from build123d import *

# Parameters (mm, degrees)
SKETCH8_R           = 2.275
BOSS_EXTRUDE4_DEPTH = 4
SKETCH9_W           = 5
SKETCH9_H           = 6
BOSS_EXTRUDE5_DEPTH = 0.75
SKETCH10_R          = 1
BOSS_EXTRUDE6_DEPTH = 3
CUT_EXTRUDE2_DEPTH  = 1.5


with BuildPart() as part:
    # Sketch8 → Boss-Extrude4 (new body)
    with BuildSketch(Plane(origin=(0, 0, 0), x_dir=(1, 0, 0), z_dir=(0, 1, 0))):
        Circle(SKETCH8_R)
    extrude(amount=BOSS_EXTRUDE4_DEPTH)

    # Sketch9 → Boss-Extrude5 (add)
    with BuildSketch(Plane(origin=(0, 4, 0), x_dir=(1, 0, 0), z_dir=(0, 1, 0))):
        Rectangle(SKETCH9_W, SKETCH9_H)
    extrude(amount=BOSS_EXTRUDE5_DEPTH)

    # Sketch10 → Boss-Extrude6 (add, symmetric)
    with BuildSketch(Plane.XY):
        with BuildLine():
            Line((-2.896323692, 6.218137436), (-2.5, 4.75))
            Line((-2.5, 4.75), (2.5, 4.75))
            Line((2.5, 4.75), (2.896323692, 6.218137436))
            ThreePointArc((2.896323692, 6.218137436), (0, 10), (-2.896323692, 6.218137436))
        make_face()
        with Locations((0, 7)):
            Circle(SKETCH10_R, mode=Mode.SUBTRACT)
    extrude(amount=BOSS_EXTRUDE6_DEPTH, both=True)

    # Sketch11 → Cut-Extrude2 (cut, symmetric)
    with BuildSketch(Plane.XY):
        with BuildLine():
            Line((-0.119661192, 4.803256683), (-17.5, 5.75))
            Line((-17.5, 5.75), (-17.5, 11.234268724))
            Line((-17.5, 11.234268724), (17.5, 11.234268724))
            Line((17.5, 11.234268724), (17.5, 5.75))
            Line((17.5, 5.75), (0.119661192, 4.803256683))
            ThreePointArc((0.119661192, 4.803256683), (0, 4.8), (-0.119661192, 4.803256683))
        make_face()
    extrude(amount=CUT_EXTRUDE2_DEPTH, both=True, mode=Mode.SUBTRACT)


solid = part.part
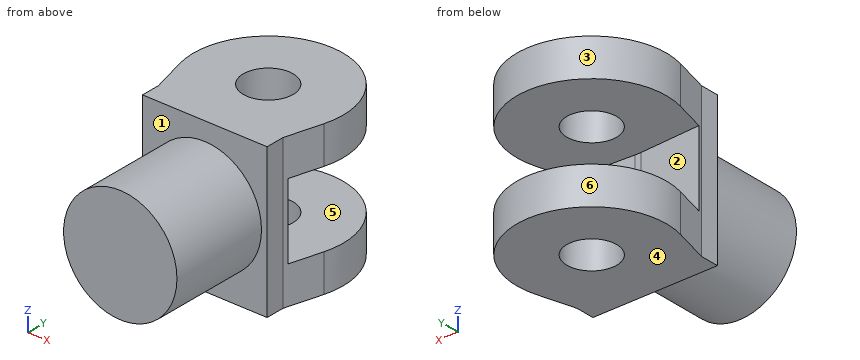
Read the model definition and answer for the solid it produces. Units are mm, in the model's axes. Face numbers are marked on the shaded views. A direction names the side the tool comes from. Coordinates: 2 decimals unless noted, no trailing zeros. Write each loop counter-clockwise with the first axis right and the second up, starting at its lowest first coordinate (ties: lowest second). Pieces come first, ordered by that corner, then holes. Notation, with made-up numbers: (86, 30) - (99, 30) arc R12 ccw to (99, 40) - close; hole circle Ø4 at (53, 34.25). An arc over 180 degrees is marked (long way). One line per question, with ' | ' between items.
Q1. Find section B-B, the plane x = 0. Write down the section's boundary in (y, z) (3 decimals).
Result set:
outline: (0, -2.275) - (4, -2.275) - (4, -3) - (6, -3) - (6, -1.5) - (4.8, -1.5) - (4.8, 1.5) - (6, 1.5) - (6, 3) - (4, 3) - (4, 2.275) - (0, 2.275) - close; (8, -3) - (10, -3) - (10, -1.5) - (8, -1.5) - close; (8, 1.5) - (10, 1.5) - (10, 3) - (8, 3) - close
Q2. Find section C-C, the plane z = 0. Write down the section's boundary in (x, y) (3 decimals).
Result set:
outline: (-2.55, 4.936) - (-2.5, 4.75) - (-2.5, 4) - (-2.275, 4) - (-2.275, 0) - (2.275, 0) - (2.275, 4) - (2.5, 4) - (2.5, 4.75) - (2.55, 4.936) - (0.12, 4.803) arc R2.2 cw to (-0.12, 4.803) - close
Q3. Each of these flat-tipped pins is pushed along its axis until it touches: P1, Ø3, axis at y = 2, z = 0.5, coming from the -X side (3 decimals); P2, Ø1.2, axis at x = 0, y = 7, coming from the +Z side; P3, Ø0.8, axis at y = 4.5, z = -1, coming from the -X side. Where does it stop, or does it pass through?
Result set:
P1: x = -2.275 | P2: through | P3: x = -2.54
Q4. Find section D-D, the plane y = 9. Write down the section's boundary in (x, z), plus the area to 3 significant figures.
Result set:
outline: (-2.24, -3) - (2.24, -3) - (2.24, -1.5) - (-2.24, -1.5) - close; (-2.24, 1.5) - (2.24, 1.5) - (2.24, 3) - (-2.24, 3) - close | area: 13.4 mm^2
Q5. For the marked faces 1, 2 and 3, determine the directions among +Z, -Z, +X, -X, +Y, -Y from which every point of the face is accessible in a straight line to the end or side of a thin tool.
Result set:
face 1: -Y | face 2: +Y | face 3: +Z, -Z
Q6. Determine the mould class of the marked faces 4, 5 and 6 for opening direction Z: +Z half, -Z half, draft (parallel to the pull), parting line (faces both ways), or undercut.
Result set:
face 4: -Z half | face 5: undercut | face 6: draft
Q7. Consider L1, parallel to X at y = 7, z = 2.6; L2, parallel to Y at x = 0, z = -1.85; L3, parallel to Y at x = 0, z = -2.45. Determine where each line is inside the solid, lowest interval first. Write a range as [from, to].
Result set:
L1: [-3, -1], [1, 3] | L2: [0, 6], [8, 10] | L3: [4, 6], [8, 10]
Q8. Find section A-A, the plane y = 7. Write down the section's boundary in (x, z), plus the area to 3 significant figures.
Result set:
outline: (-3, -3) - (-1, -3) - (-1, -1.5) - (-3, -1.5) - close; (-3, 1.5) - (-1, 1.5) - (-1, 3) - (-3, 3) - close; (1, -3) - (3, -3) - (3, -1.5) - (1, -1.5) - close; (1, 1.5) - (3, 1.5) - (3, 3) - (1, 3) - close | area: 12.0 mm^2
